Drawing for the job (mm, zero at the part's lowest x, y, z). A direction names the side the tool comes from. Coordinates: 2 decimals unless noted, no trailing zeros. Loops run counter-clockwise (first coordinate to the right, second up) from the corner with the lowest first, then second, coordinate; pieces in that order, holes last.
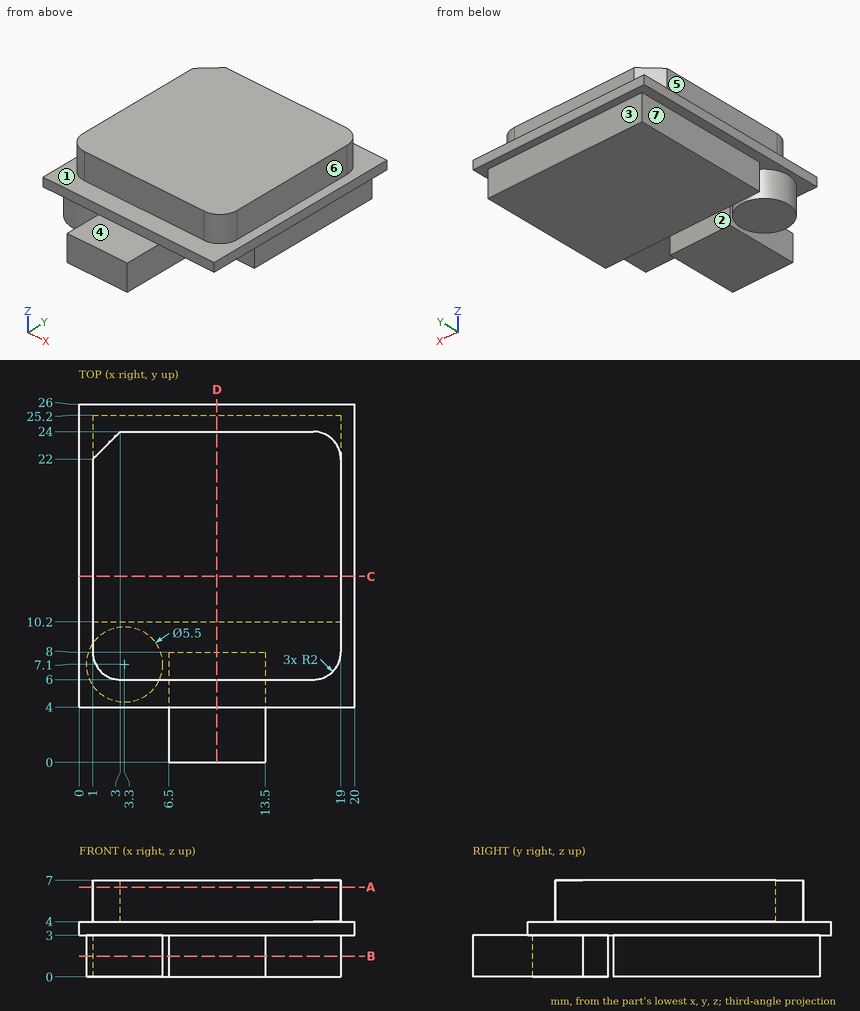
Q1. Mould opens along Y. For the marked faces 1, 2 and 3 say: released by +Y, released by -Y, zero draft, split by the parting line, or undercut.
Q2. Probe line 1 (Y direction, x = 10.5, z = 1.75); line 2 (Y direction, x = 5.5, z = 4.25); line 3 (X direction, y = 9.25, z = 5.5). List the from-to ranges inside material, lowest first.
Q3. Saw through at D-D (x = 10). List the corners of the cut face in (y, z), plus the area to 3 significant figures.
Q4. Saw through at B-B (z = 1.5). List the corners of the cut face in (x, y).
Q5. Saw through at A-A (z = 6.5). List the corners of the cut face in (x, y).
Q6. Saw through at C-C (y = 13.5). List the corners of the cut face in (x, z).
Q7. Tool access for the marked faces 4, 5, 6 and 7: list every direction of +Z, -Z, +X, -X, +Y, -Y with a clear straight run to the whole face (end or side of a thin tool).
Q8. Drop flat-ended pins along their axis: P1, Ø2.5, axis at y = 3, z = 1.5, coming from the -X side; P2, Ø2.5, axis at y = 19.5, z = 1, coming from the -X side; P3, Ø3.5, axis at y = 6, z = 1, coming from the +X side. Give the stop position or say it passes through.
Checked values:
1. face 1: zero draft
1. face 2: undercut
1. face 3: released by +Y
2. line 1: y = 0 to 8, 10.2 to 25.2
2. line 2: y = 6 to 24
2. line 3: x = 1 to 19
3. outline: (0, 0) - (8, 0) - (8, 3) - (10.2, 3) - (10.2, 0) - (25.2, 0) - (25.2, 3) - (26, 3) - (26, 4) - (24, 4) - (24, 7) - (6, 7) - (6, 4) - (4, 4) - (4, 3) - (0, 3) - close
3. area: 145 mm2
4. outline: circle Ø5.5 at (3.3, 7.1); (1, 10.2) - (19, 10.2) - (19, 25.2) - (1, 25.2) - close; (6.5, 0) - (13.5, 0) - (13.5, 8) - (6.5, 8) - close
5. outline: (1, 8) arc R2 ccw to (3, 6) - (17, 6) arc R2 ccw to (19, 8) - (19, 22) arc R2 ccw to (17, 24) - (3, 24) - (1, 22) - close
6. outline: (0, 3) - (1, 3) - (1, 0) - (19, 0) - (19, 3) - (20, 3) - (20, 4) - (19, 4) - (19, 7) - (1, 7) - (1, 4) - (0, 4) - close
7. face 4: +Z, +X, -X, -Y
7. face 5: +Z, -X, +Y, -Y
7. face 6: +Z, +X, +Y, -Y
7. face 7: -Z, -X, +Y
8. P1: stops at x = 6.5
8. P2: stops at x = 1
8. P3: stops at x = 13.5
